Work out the finished part from the listing and answer in its coordinate system (mm). Coordinates: 2 decimals unless noted, no trailing zeros. Order: outer loops, then holes, each group sorted by start corner. A loop starts at its lowest first (then second) coordinate and runs counter-clockwise, first axis right, second up. Notation, with made-up numbers: M 5.5,81 L 14.5,81 A19 ccw 14.5,90 Z; hole C 43.25,70.5 d8. An arc over 180 degrees is marked long. Write item = value, one per line. Start each with the question number.
Q1. Find section C-C on x = 6.5. Give the vertices of the cut face in (y, z), and give its area (3 significant figures).
Q2. Find section B-B on z = 126.5. Give the vertices of the cut face in (x, y), and give its area (3 significant figures).
Q3. Each of these flat-tipped pins is pushed along its axis until it touches: P1, Ø0.9, axis at y = 2, z = -9, coming from the -X side; P2, Ø0.9, axis at y = 1.5, z = 190.5, coming from the -X side; P3, Ø1.5, axis at y = 2, z = 110, coming from the -X side. Where does it stop, or does it pass through?
Q4. Straight lines are drawn through the part: line 1 along Z through (x, y) = (4.5, 1.6); line 2 along X through (y, z) = (0.55, 175); line 3 along X through (y, z) = (2.4, 34). For each, find the intervals that lie inside material, in ascending order.
Q5. Find section A-A on y = 2.45. Give the vertices of the cut face in (x, z).
```python
from build123d import *

# Parameters (mm, degrees)
SALIENTE_EXTRUIR1_DEPTH = 3


with BuildPart() as part:
    # Croquis1 → Saliente-Extruir1 (new body)
    with BuildSketch(Plane(origin=(0, 0, 0), x_dir=(1, 0, 0), z_dir=(0, 1, 0))):
        with BuildLine():
            Line((0, 7.786096257), (0, 0))
            Line((0, 0), (0, -0.213903743))
            Line((0, -0.213903743), (3, -0.213903743))
            Line((3, -0.213903743), (3, -2.106951872))
            Line((3, -2.106951872), (7.35828877, -2.106951872))
            Line((7.35828877, -2.106951872), (28.573593129, -2.106951872))
            ThreePointArc((28.573593129, -2.106951872), (54.330952442, -12.77599943), (65, -38.533358743))
            Line((65, -38.533358743), (65, -117.736951872))
            Line((65, -117.736951872), (65, -188.736951872))
            Line((65, -188.736951872), (67, -188.736951872))
            Line((67, -188.736951872), (67, -191.736951872))
            Line((67, -191.736951872), (75, -191.736951872))
            Line((75, -191.736951872), (75, -188.736951872))
            Line((75, -188.736951872), (77, -188.736951872))
            Line((77, -188.736951872), (77, -38.533358743))
            ThreePointArc((77, -38.533358743), (62.816233816, -4.290718056), (28.573593129, 9.893048128))
            Line((28.573593129, 9.893048128), (3, 9.893048128))
            Line((3, 9.893048128), (3, 8))
            Line((3, 8), (0, 8))
            Line((0, 8), (0, 7.786096257))
        make_face()
    extrude(amount=SALIENTE_EXTRUIR1_DEPTH)


solid = part.part
```
Findings below:
q1.outline = M 0,-9.89 L 3,-9.89 L 3,2.11 L 0,2.11 Z
q1.area = 36.0 mm^2
q2.outline = M 65,0 L 77,0 L 77,3 L 65,3 Z
q2.area = 36.0 mm^2
q3.P1 = 3
q3.P2 = 67
q3.P3 = 65
q4.line_1 = -9.89 to 2.11
q4.line_2 = 65 to 77
q4.line_3 = 64.72 to 76.79
q5.outline = M 0,-8 L 3,-8 L 3,-9.89 L 28.57,-9.89 A48.43 ccw 77,38.53 L 77,188.74 L 75,188.74 L 75,191.74 L 67,191.74 L 67,188.74 L 65,188.74 L 65,38.53 A36.43 cw 28.57,2.11 L 3,2.11 L 3,0.21 L 0,0.21 Z
